Work out the finished part from the listing and answer in its coordinate system (mm). A direction names the side the tool comes from. Give positions to 0.01 mm unless a question says otherwise; leave off trailing zeros. Loops run counter-clockwise (first coordinate to the right, second up) from the corner with the lowest first, then second, coordinate; pieces in that order, holes last.
from build123d import *

# Parameters (mm, degrees)
ESQUISSE1_W             = 10
ESQUISSE1_H             = 8.4
BOSS_EXTRU_1_DEPTH      = 12.2
ENL_V_MAT_EXTRU_1_DEPTH = 8.5
ESQUISSE3_W             = 4.3
ESQUISSE3_H             = 0.5
ENL_V_MAT_EXTRU_2_DEPTH = 11
ESQUISSE4_R             = 0.6
BOSS_EXTRU_2_DEPTH      = 4
BOSS_EXTRU_2_DEPTH_BACK = 11.5
CHANFREIN1_SIZE         = 0.2
CHANFREIN1_SIZE2        = 0.746410162
CHANFREIN1_PART_2_SIZE  = 0.2
CHANFREIN1_PART_2_SIZE2 = 0.746410162
CHANFREIN2_SIZE         = 0.2
ESQUISSE5_R             = 1.1
BOSS_EXTRU_3_DEPTH      = 0.6


with BuildPart() as part:
    # Esquisse1 → Boss.-Extru.1 (new body)
    with BuildSketch(Plane.XY):
        with Locations((5, 4.2)):
            Rectangle(ESQUISSE1_W, ESQUISSE1_H)
    extrude(amount=BOSS_EXTRU_1_DEPTH)

    # Esquisse2 → Enlèv. mat.-Extru.1 (cut)
    with BuildSketch(Plane.XY.offset(12.2)):
        with BuildLine():
            Line((0, 1.4), (0, 6.9))
            Line((0, 6.9), (10, 6.9))
            Line((10, 6.9), (10, 1.4))
            Line((10, 1.4), (9.34, 1.4))
            ThreePointArc((9.34, 1.4), (7.54, 0.8), (5.74, 1.4))
            Line((5.74, 1.4), (4.26, 1.4))
            ThreePointArc((4.26, 1.4), (2.46, 0.8), (0.66, 1.4))
            Line((0.66, 1.4), (0, 1.4))
        make_face()
    extrude(amount=-ENL_V_MAT_EXTRU_1_DEPTH, mode=Mode.SUBTRACT)

    # Esquisse3 → Enlèv. mat.-Extru.2 (cut, through all)
    with BuildSketch(Plane.ZY):
        with Locations((6.85, 8.15)):
            Rectangle(ESQUISSE3_W, ESQUISSE3_H)
        Polygon((12.2, 8.4), (9.2, 8.4), (12.2, 8.05), align=None)
        Polygon((12.2, 7.25), (12.2, 6.9), (9.2, 6.9), align=None)
    extrude(amount=-ENL_V_MAT_EXTRU_2_DEPTH, mode=Mode.SUBTRACT)

    # Esquisse4 → Boss.-Extru.2 (add, two sides)
    with BuildSketch(Plane(origin=(0, 0, 0), x_dir=(-1, 0, 0), z_dir=(0, 0, -1))) as boss_extru_2_sk:
        with Locations((-7.54, 3.75)):
            Circle(ESQUISSE4_R)
        with Locations((-2.46, 3.75)):
            Circle(ESQUISSE4_R)
    extrude(amount=BOSS_EXTRU_2_DEPTH)
    extrude(boss_extru_2_sk.sketch, amount=-BOSS_EXTRU_2_DEPTH_BACK)

    # Chanfrein1
    chanfrein1_edges = [part.edges().sort_by_distance(p)[0] for p in [
        (8.14, 3.75, 11.5),
    ]]
    chanfrein1_side = [part.faces().sort_by_distance(p)[0] for p in [
        (7.54, 3.75, 11.5),
    ]]
    chamfer(chanfrein1_edges, length=CHANFREIN1_SIZE, length2=CHANFREIN1_SIZE2, reference=chanfrein1_side[0])

    # Chanfrein1 part 2
    chanfrein1_part_2_edges = [part.edges().sort_by_distance(p)[0] for p in [
        (3.06, 3.75, 11.5),
    ]]
    chanfrein1_part_2_side = [part.faces().sort_by_distance(p)[0] for p in [
        (2.46, 3.75, 11.5),
    ]]
    chamfer(chanfrein1_part_2_edges, length=CHANFREIN1_PART_2_SIZE, length2=CHANFREIN1_PART_2_SIZE2, reference=chanfrein1_part_2_side[0])

    # Chanfrein2
    chanfrein2_edges = [part.edges().sort_by_distance(p)[0] for p in [
        (8.14, 3.75, -4),
        (3.06, 3.75, -4),
    ]]
    chamfer(chanfrein2_edges, length=CHANFREIN2_SIZE)

    # Esquisse5 → Boss.-Extru.3 (add)
    with BuildSketch(Plane.XY.offset(3.7)):
        with Locations((2.46, 3.75)):
            Circle(ESQUISSE5_R)
        with Locations((7.54, 3.75)):
            Circle(ESQUISSE5_R)
    extrude(amount=BOSS_EXTRU_3_DEPTH)


solid = part.part
Item 1: Determine the mould class of faces 5 (the face through (5, 1.4, 8)), 6 (the face through (0, 4, 3)), 7 (the face through (4.93, 8.227, 10.679)), 8 (the face through (6.968, 3.93, -1.873)) for opening direction Y: released by +Y, released by -Y, zero draft, split by the parting line, or undercut.
Item 2: Find section C-C, the plane x = 9. Write down the section's boundary in (y, z).
Item 3: Find section B-B, the plane z = -1.25. Write down the section's boundary in (x, y).
Item 4: Find section D-D, the plane x = 3.75. Write down the section's boundary in (y, z), plus the area to 3 significant figures.
Item 5: For faces 1 (the face through (5, 4, 3.7)), 2 (the face through (5, 7.9, 7)), 3 (the face through (4.93, 7.073, 10.679)), 4 (the face through (2.137, 4.256, -1.873)), determine the directions among +Z, -Z, +X, -X, +Y, -Y from which every point of the face is accessible in a straight line to the end or side of a thin tool.
Item 6: Flat-ended cylindrical pins translate along their axes: pin 1 Ø1 at (y, z) = (3.5, 8.5) entering from -X; pin 2 Ø1.8 at (x, y) = (7, 4) entering from +Z; pin 3 Ø3.5 at (x, z) = (3.5, 7) entering from +Y. Find the tip coordinate at first contact, or state that the pin passes through.
Item 7: Consider line 1 (Y direction, x = 7.5, z = 7.25); line 2 (Y direction, x = 3, z = 5.75); line 3 (Z direction, x = 2, y = 3). Determine where each line is inside the solid, lowest interval first.
Ans:
1. face 5: undercut
1. face 6: zero draft
1. face 7: released by +Y
1. face 8: split by the parting line
2. outline: (0, 0) - (8.4, 0) - (8.4, 4.7) - (7.9, 4.7) - (7.9, 9) - (8.4, 9) - (8.4, 9.2) - (8.05, 12.2) - (7.25, 12.2) - (6.9, 9.2) - (6.9, 3.7) - (1.18, 3.7) - (1.18, 12.2) - (0, 12.2) - close
3. outline: circle Ø1.2 at (2.46, 3.75); circle Ø1.2 at (7.54, 3.75)
4. outline: (0, 0) - (8.4, 0) - (8.4, 4.7) - (7.9, 4.7) - (7.9, 9) - (8.4, 9) - (8.4, 9.2) - (8.05, 12.2) - (7.25, 12.2) - (6.9, 9.2) - (6.9, 3.7) - (1.09, 3.7) - (1.09, 12.2) - (0, 12.2) - close
4. area: 49.9 mm2
5. face 1: +Z
5. face 2: +X, -X, +Y
5. face 3: +Z, +X, -X
5. face 4: -Z
6. pin 1: stops at x = 1.86
6. pin 2: stops at z = 11.5
6. pin 3: stops at y = 7.9
7. line 1: y = 0 to 0.8, 3.15 to 4.35, 6.9 to 7.9
7. line 2: y = 0 to 0.85, 3.49 to 4.01, 6.9 to 7.9
7. line 3: z = 0 to 4.3
